from build123d import *

# Parameters (mm, degrees)
SKETCH_1_W             = 120
SKETCH_1_H             = 45
SKETCH_1_R             = 10.75
EXTRUDE_1_DEPTH        = 50
HOLE_WIZARD_M6_1_D     = 5.5
HOLE_WIZARD_M6_1_DEPTH = 15
HOLE_WIZARD_M6_1_TIP   = 1.652366702


with BuildPart() as part:
    # 草图1 → 凸台-拉伸1 (new body)
    with BuildSketch(Plane(origin=(0, 0, 0), x_dir=(1, 0, 0), z_dir=(0, 1, 0))):
        Rectangle(SKETCH_1_W, SKETCH_1_H)
        with Locations(Location((-35, 0, 0), (0, 0, 270))):
            Circle(SKETCH_1_R, mode=Mode.SUBTRACT)
        with Locations(Location((35, 0, 0), (0, 0, 90))):
            Circle(SKETCH_1_R, mode=Mode.SUBTRACT)
    extrude(amount=EXTRUDE_1_DEPTH)

    # M6 螺纹孔1
    with Locations(Plane(origin=(-48, 43, 22.5), x_dir=(1, 0, 0), z_dir=(0, 0, 1))):
        with Locations((0, 0), (0, -36)):
            Hole(HOLE_WIZARD_M6_1_D / 2, depth=HOLE_WIZARD_M6_1_DEPTH)
            with Locations((0, 0, -(HOLE_WIZARD_M6_1_DEPTH + HOLE_WIZARD_M6_1_TIP / 2))):  # 118° drill point
                Cone(0, HOLE_WIZARD_M6_1_D / 2, HOLE_WIZARD_M6_1_TIP, mode=Mode.SUBTRACT)


solid = part.part
Model file for the job. Use its own axes, mm. A direction names the side the tool comes from. Give positions to 0.01 mm unless a question says otherwise; leave off trailing zeros. Order: outer loops, then holes, each group sorted by start corner. A loop starts at its lowest first (then second) coordinate and runs counter-clockwise, first axis right, second up. Notation, with made-up numbers: (-16, -20) - (2, -20) arc R35 ccw to (2, 13) - close; hole circle Ø1 at (74.5, -23). An arc over 180 degrees is marked (long way). One line per item, written item: value.
Item 1: Pin check, flat tip, straight feed: pin 1 Ø13 at (x, z) = (35, 0) entering from +Y. Stop position of the tip, or through.
Response values:
pin 1: through
Item 2: Slice it at A-A (x = -35). List the corners of the cut face in (y, z), then the cut area to 4 significant figures.
Response values:
outline: (0, -22.5) - (50, -22.5) - (50, -10.75) - (0, -10.75) - close; (0, 10.75) - (50, 10.75) - (50, 22.5) - (0, 22.5) - close
area: 1,175 mm2
Item 3: Slice it at B-B (y = 39). List the corners of the cut face in (x, z).
Response values:
outline: (-60, -22.5) - (60, -22.5) - (60, 22.5) - (-60, 22.5) - close; hole circle Ø21.5 at (-35, 0); hole circle Ø21.5 at (35, 0)
Item 4: Tool access for faces 1 (the cylindrical face through (-45.973, 44.859, 14.895)), 2 (the cylindrical face through (24.34, 24.65, 1.4)): list every direction of +Z, -Z, +X, -X, +Y, -Y with a clear straight run to the whole face (end or side of a thin tool).
Response values:
face 1: +Z
face 2: +Y, -Y
Item 5: Slice it at C-C (x = 32.5). List the corners of the cut face in (y, z).
Response values:
outline: (0, -22.5) - (50, -22.5) - (50, -10.46) - (0, -10.46) - close; (0, 10.46) - (50, 10.46) - (50, 22.5) - (0, 22.5) - close
Item 6: Two-plate mould, pull along X, no slides. Class faces 3 (the cylindrical face through (-45.253, 7.121, 14.895)), 4 (the flat face through (-1, 0, 0)), 5 (the flat face through (60, 25, 0)): released by +X, released by -X, zero draft, split by the parting line, or undercut.
Response values:
face 3: undercut
face 4: zero draft
face 5: released by +X
Item 7: Wall check: line 1 (X direction, y = 21, z = 0); line 2 (Y direction, x = -48, z = 16); line 3 (X direction, y = 15.5, z = 9). Give the ranges that are in metal, low to high.
Response values:
line 1: -60 to -45.75, -24.25 to 24.25, 45.75 to 60
line 2: 0 to 4.25, 9.75 to 40.25, 45.75 to 50
line 3: -60 to -40.88, -29.12 to 29.12, 40.88 to 60
Item 8: Slice it at D-D (y = 44.5). Give the number of separate pieces and of enclosed holes in the cut face, then the cut area to 3 significant figures.
Response values:
separate pieces: 1
enclosed holes: 2
area: 4,600 mm2
